Part model, mm, in its own coordinate system. Face numbers are marked on the shaded views. A direction names the side the tool comes from. Round coordinates to 2 decimals unless told otherwise and drop trailing zeros. Order: outer loops, then holes, each group sorted by start corner. A loop starts at its lowest first (then second) coordinate and runs counter-clockwise, first axis right, second up. Notation, with made-up numbers: (57.25, 64) -> (91.25, 64) arc R29 cw to (91.25, 86) -> close; hole circle Ø5 at (53, 30.25). An arc over 180 degrees is marked (long way). Use CSV: the item, a comma, the result in double quotes.
Autodesk Fusion 360 part; units mm, degrees
sketch "Base" plane through (0, 0, 0) normal (0, 1, 0) x (1, 0, 0)
  circle A0 centre (0, 0) radius 7
  dimension "d1" = 14
extrude "Extrude1" add sketch "Base" along normal blind 4
sketch "Pin" plane through (0, 4, 0) normal (0, 1, 0) x (-1, 0, 0)
  circle A0 centre (0, 0) radius 7
  circle A1 centre (0, 0) radius 3.9
  dimension "d4" = 7.8
extrude "Extrude2" add sketch "Pin" along normal blind 25 contours A1
hole "Hole1" at (-0.0382, 0, -0.0078) direction (0, 1, 0) diameter 2 end through all
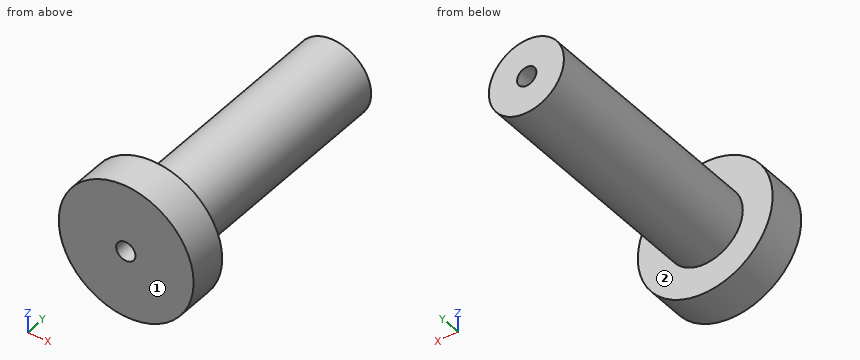
(1) Drop flat-ended pins along their axis: P1, Ø3, axis at x = -4, y = 26, coming from the +Z side; P2, Ø8, axis at y = 18.5, z = 2, coming from the +X side; P3, Ø1.5, axis at x = -4, y = 20.5, coming from the +Z side. Give the stop position or say it passes through.
Reply:
P1,"z = 2.99"
P2,"x = 3.9"
P3,"z = 2.16"
(2) Cut at B-B, the plane z = 0. Give the cut face in (x, y), then the cut area to 3 significant figures.
Reply:
outline,"(-7, 0) -> (-1.04, 0) -> (-1.04, 29) -> (-3.9, 29) -> (-3.9, 4) -> (-7, 4) -> close; (0.96, 0) -> (7, 0) -> (7, 4) -> (3.9, 4) -> (3.9, 29) -> (0.96, 29) -> close"
area,"193 mm2"
(3) Cut at C-C, the plane x = -3. Give the cut face in (y, z).
Reply:
outline,"(0, -6.32) -> (4, -6.32) -> (4, -2.49) -> (29, -2.49) -> (29, 2.49) -> (4, 2.49) -> (4, 6.32) -> (0, 6.32) -> close"
(4) Cut at A-A, the plane x = -0.75. Give the cut face in (y, z).
Reply:
outline,"(0, -6.96) -> (4, -6.96) -> (4, -3.83) -> (29, -3.83) -> (29, -0.71) -> (0, -0.71) -> close; (0, 0.69) -> (29, 0.69) -> (29, 3.83) -> (4, 3.83) -> (4, 6.96) -> (0, 6.96) -> close"
(5) Which spindle directions (+Z, -Z, +X, -X, +Y, -Y) get a long thin tool onto all of the face, cutting with end or side? Do the marked faces 1 and 2. Say none if no direction does.
Reply:
face 1,"+Z, -Z, +X, -X, -Y"
face 2,"+Y"
(6) Probe probe 1 along Z at (x, y) = (0, 19); probe 2 along Y at (x, z) = (0, -6); probe 3 along Z at (x, y) = (0.75, 5.5). List the from-to ranges inside material, lowest first. Write a range as [from, to].
Reply:
probe 1,"[-3.9, -1.01], [0.99, 3.9]"
probe 2,"[0, 4]"
probe 3,"[-3.83, -0.62], [0.61, 3.83]"
(7) Cut at D-D, the plane y = 25.5. Give the cut face in (x, z).
Reply:
outline,"circle Ø7.8 at (0, 0); hole circle Ø2 at (-0.04, -0.01)"
